Geometry: final body of the model. Coordinates: model frame, mm. A direction names the side the tool comes from. Give positions to 0.01 mm unless a question says otherwise; leave off trailing zeros. Loops run counter-clockwise (first coordinate to the right, second up) from the corner with the lowest first, then second, coordinate; pieces in that order, holes last. Notation, with made-up numbers: (86, 78.5) - (110, 78.5) arc R25 ccw to (110, 92.5) - close; hole circle Ø5 at (-9.5, 34.25). An arc over 180 degrees is marked (long way). Use one line per item in the form item = value.
```python
from build123d import *

# Parameters (mm, degrees)
SKETCH023_R  = 1.75
PAD012_DEPTH = 3
SKETCH024_W  = 16.5
SKETCH024_H  = 38
PAD013_DEPTH = 21.6


with BuildPart() as part:
    # Sketch021 → Revolution005 (revolve)
    with BuildSketch(Plane.XY):
        Polygon((0, 0), (0, -32), (12, -32), (12, 0), (30, 0), (27.75, 10), (0, 10), align=None)
    revolve(axis=Axis((0, 0, 0), (0, 1, 0)))

    # Sketch023 → Pad012 (new body)
    with BuildSketch(Plane.XZ):
        with Locations((18.75, 0)):
            Circle(SKETCH023_R)
        with Locations((-18.75, 0)):
            Circle(SKETCH023_R)
    extrude(amount=PAD012_DEPTH)

    # Sketch024 (on Face1 of Pad012) → Pad013 (join)
    with BuildSketch(Plane.XZ.offset(32)):
        with Locations((0, 4.5)):
            Rectangle(SKETCH024_W, SKETCH024_H)
    extrude(amount=PAD013_DEPTH)


solid = part.part
```
(1) Cut plane B-B (z = 0). Return the cut outline in (x, y).
Solution:
outline = (-30, 0) - (-20.5, 0) - (-20.5, -3) - (-17, -3) - (-17, 0) - (-12, 0) - (-12, -32) - (-8.25, -32) - (-8.25, -53.6) - (8.25, -53.6) - (8.25, -32) - (12, -32) - (12, 0) - (17, 0) - (17, -3) - (20.5, -3) - (20.5, 0) - (30, 0) - (27.75, 10) - (-27.75, 10) - close
(2) Access query for faces 4 (the face through (0, -32, -13)), 5 (the face through (-19, -3, 0)), 6 (the face through (0, 0, 13)). Directions: +Z, -Z, +X, -X, +Y, -Y. A direction counts if a zero-diameter tool reaches every point of the face in a straight line with its end or side. Return the directions, or none.
Solution:
face_4 = -Z
face_5 = +Z, -Z, -X, -Y
face_6 = none
(3) Cut plane A-A (x = 0). Return the cut outline in (y, z), plus the area to 3 significant figures.
Solution:
outline = (-53.6, -14.5) - (-32, -14.5) - (-32, -12) - (0, -12) - (0, -30) - (10, -27.75) - (10, 27.75) - (0, 30) - (0, 12) - (-32, 12) - (-32, 23.5) - (-53.6, 23.5) - close
area = 2,170 mm2
(4) Pull-direction query (X, two-part tool) for faces 1 (the face through (10, -32, 0)), 2 (the face through (17, -1, 0)), 3 (the face through (8.25, -43, 4)); classes: released by +X, released by -X, zero draft, split by the parting line, or undercut.
Solution:
face_1 = zero draft
face_2 = undercut
face_3 = released by +X
(5) Pin query (flat end, axial travel): P1, Ø8, axis at x = -0.5, y = -48, coming from the -Z side; P2, Ø1.1, axis at x = -9.5, z = 0, coming from the -Y side; P3, Ø3, axis at x = 18.5, z = -0.5, coming from the -Y side. Return the tip coordinate at first contact, or that it passes through.
Solution:
P1 = -14.5
P2 = -32
P3 = -3
(6) Cut plane D-D (y = -25.5). Return the cut outline in (x, z).
Solution:
outline = circle Ø24 at (0, 0)
(7) Material intervals for L1, parallel to Y at x = -14, z = 21.5; L2, parallel to Z at x = 0, y = -13.5; L3, parallel to Z at x = 3, y = -47, sorted ascending. Write a range as from..to.
Solution:
L1 = 0..10
L2 = -12..12
L3 = -14.5..23.5
(8) Cut plane C-C (y = -40). Return the cut outline in (x, z), plus the area to 3 significant figures.
Solution:
outline = (-8.25, -14.5) - (8.25, -14.5) - (8.25, 23.5) - (-8.25, 23.5) - close
area = 627 mm2
